Part model, mm, in its own coordinate system. Face numbers are marked on the shaded views. A direction names the side the tool comes from. Round coordinates to 2 decimals unless told otherwise and drop trailing zeros. Order: outer loops, then holes, each group sorted by start corner. A loop starts at its lowest first (then second) coordinate and runs counter-clockwise, first axis right, second up. Notation, with made-up numbers: M 80,34 L 109,34 A16 cw 109,62 Z; hole C 35,-7 d7. An arc over 180 degrees is marked long. Write each question's results on one line, items separated by ' | '. Start each with the question number.
1. Band-saw the part on B-B, the plane z = 0. List the corners of the cut face in (x, y).
2. Drop flat-ended pins along their axis: pin 1 Ø1.3 at (y, z) = (4.5, -1) entering from +X; pin 2 Ø3.5 at (x, z) = (-36.068, -8.128) entering from -Y; pin 3 Ø1.5 at (x, y) = (29, 3.5) entering from -Z; pin 4 Ø3 at (x, z) = (-25.5, 0) entering from +Y. Give the stop position or say it passes through.
3. Band-saw the part on A-A, the plane x = 0. List the corners of the cut face in (y, z).
4. Band-saw the part on C-C, the plane x = -18. List the corners of the cut face in (y, z).
5. Two-plate mould, pull along X, no slides. Class the marked faces 1, 2 and 3: +X half, -X half, draft (parallel to the pull), parting line (faces both ways), or undercut.
6. Which spindle directions (+Z, -Z, +X, -X, +Y, -Y) get a long thin tool onto all of the face, cutting with end or side? Do the marked faces 4 and 5. Say none if no direction does.
7. Band-saw the part on D-D, the plane y = 2.25. List the corners of the cut face in (x, z).
8. Probe L1, parallel to X at y = 4.5, z = -7; L2, parallel to X at y = 0.5, z = -7; L3, parallel to Z at x = 27.5, y = 5.75. List the from-to ranges inside material, lowest first. Write a range as [from, to].
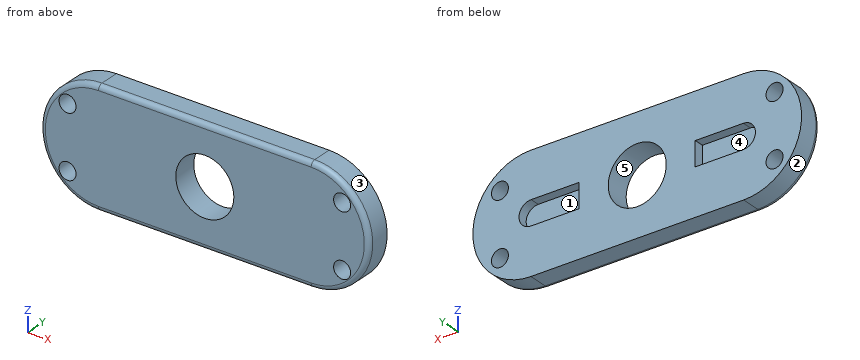
```python
from build123d import *

# Parameters (mm, degrees)
BOSS_EXTRUDE1_DEPTH = 6.35
CUT_EXTRUDE1_DEPTH  = 2.54
SKETCH3_R           = 7.62
CUT_EXTRUDE2_DEPTH  = 47.228697797
FILLET1_R           = 1.27
SKETCH4_R           = 2.23393
CUT_EXTRUDE3_DEPTH  = 47.228697923


with BuildPart() as part:
    # Sketch1 → Boss-Extrude1 (new body)
    with BuildSketch(Plane(origin=(0, 0, 0), x_dir=(1, 0, 0), z_dir=(0, 1, 0))):
        with BuildLine():
            Line((27.94, 15.24), (-27.94, 15.24))
            ThreePointArc((-27.94, 15.24), (-43.18, 0), (-27.94, -15.24))
            Line((-27.94, -15.24), (27.94, -15.24))
            ThreePointArc((27.94, -15.24), (43.18, 0), (27.94, 15.24))
        make_face()
    extrude(amount=BOSS_EXTRUDE1_DEPTH)

    # Sketch2 → Cut-Extrude1 (cut)
    with BuildSketch(Plane(origin=(0, 6.35, 0), x_dir=(1, 0, 0), z_dir=(0, 1, 0))):
        with BuildLine():
            Line((-15.24, 3.063440359), (-27.882747925, 3.063440359))
            ThreePointArc((-27.882747925, 3.063440359), (-31.057747925, -0.111559641), (-27.882747925, -3.286559641))
            Line((-27.882747925, -3.286559641), (-15.24, -3.286559641))
            Line((-15.24, -3.286559641), (-15.24, 3.063440359))
        make_face()
        with BuildLine():
            Line((15.24, 3.063440359), (15.24, -3.286559641))
            Line((15.24, -3.286559641), (27.882747925, -3.286559641))
            ThreePointArc((27.882747925, -3.286559641), (31.057747925, -0.111559641), (27.882747925, 3.063440359))
            Line((27.882747925, 3.063440359), (15.24, 3.063440359))
        make_face()
    extrude(amount=-CUT_EXTRUDE1_DEPTH, mode=Mode.SUBTRACT)

    # Sketch3 → Cut-Extrude2 (cut, through all)
    with BuildSketch(Plane(origin=(0, 6.35, 0), x_dir=(1, 0, 0), z_dir=(0, 1, 0))):
        with Locations(Location((0, 0, 0), (0, 0, 270))):
            Circle(SKETCH3_R)
    extrude(amount=-CUT_EXTRUDE2_DEPTH, mode=Mode.SUBTRACT)

    # Fillet1
    fillet1_edges = [part.edges().sort_by_distance(p)[0] for p in [
        (0, 0, -15.24),
        (43.18, 0, 0),
        (0, 0, 15.24),
        (-43.18, 0, 0),
    ]]
    fillet(fillet1_edges, radius=FILLET1_R)

    # Sketch4 → Cut-Extrude3 (cut, through all)
    with BuildSketch(Plane(origin=(0, 6.35, 0), x_dir=(1, 0, 0), z_dir=(0, 1, 0))):
        with Locations(Location((-36.068, 8.128, 0), (0, 0, 270))):
            Circle(SKETCH4_R)
        with Locations(Location((-36.068, -8.128, 0), (0, 0, 270))):
            Circle(SKETCH4_R)
        with Locations(Location((36.068, 8.128, 0), (0, 0, 90))):
            Circle(SKETCH4_R)
        with Locations(Location((36.068, -8.128, 0), (0, 0, 90))):
            Circle(SKETCH4_R)
    extrude(amount=-CUT_EXTRUDE3_DEPTH, mode=Mode.SUBTRACT)


solid = part.part
```
Solution:
1) outline: M -43.18,1.27 A1.27 ccw -41.91,0 L -7.62,0 L -7.62,6.35 L -15.24,6.35 L -15.24,3.81 L -31.06,3.81 L -31.06,6.35 L -43.18,6.35 Z; M 7.62,0 L 41.91,0 A1.27 ccw 43.18,1.27 L 43.18,6.35 L 31.06,6.35 L 31.06,3.81 L 15.24,3.81 L 15.24,6.35 L 7.62,6.35 Z
2) pin 1: x = 43.18 | pin 2: through | pin 3: z = -15.24 | pin 4: y = 3.81
3) outline: M 0,-13.97 A1.27 ccw 1.27,-15.24 L 6.35,-15.24 L 6.35,-7.62 L 0,-7.62 Z; M 0,7.62 L 6.35,7.62 L 6.35,15.24 L 1.27,15.24 A1.27 ccw 0,13.97 Z
4) outline: M 0,-13.97 A1.27 ccw 1.27,-15.24 L 6.35,-15.24 L 6.35,-3.06 L 3.81,-3.06 L 3.81,3.29 L 6.35,3.29 L 6.35,15.24 L 1.27,15.24 A1.27 ccw 0,13.97 Z
5) face 1: undercut | face 2: -X half | face 3: +X half
6) face 4: +Y | face 5: +Y, -Y
7) outline: M -27.94,-15.24 L 27.94,-15.24 A15.24 ccw 27.94,15.24 L -27.94,15.24 A15.24 ccw Z; hole C -36.07,-8.13 d4.47; hole C -36.07,8.13 d4.47; hole C 0,0 d15.24; hole C 36.07,-8.13 d4.47; hole C 36.07,8.13 d4.47
8) L1: [-41.48, -38], [-34.14, -3.01], [3.01, 34.14], [38, 41.48] | L2: [-41.18, -38], [-34.14, -3.01], [3.01, 34.14], [38, 41.18] | L3: [-15.24, -3.06], [3.29, 15.24]
